from build123d import *

# Parameters (mm, degrees)
SKETCH1_R           = 1.625
SKETCH1_W           = 4
SKETCH1_H           = 10
BOSS_EXTRUDE1_DEPTH = 4


with BuildPart() as part:
    # Sketch1 → Boss-Extrude1 (new body)
    with BuildSketch(Plane(origin=(0, 0, 0), x_dir=(1, 0, 0), z_dir=(0, 1, 0))):
        Polygon((0, 0), (20, 0), (27.5, 0), (27.5, 4), (42.5, 4), (42.5, 0), (50, 0), (70, 0), (70, 26), (0, 26), align=None)
        with Locations((10, 19)):
            Circle(SKETCH1_R, mode=Mode.SUBTRACT)
        with Locations((60, 19)):
            Circle(SKETCH1_R, mode=Mode.SUBTRACT)
        with Locations((20, 16)):
            Rectangle(SKETCH1_W, SKETCH1_H, mode=Mode.SUBTRACT)
        with Locations((50, 16)):
            Rectangle(SKETCH1_W, SKETCH1_H, mode=Mode.SUBTRACT)
    extrude(amount=BOSS_EXTRUDE1_DEPTH)


solid = part.part
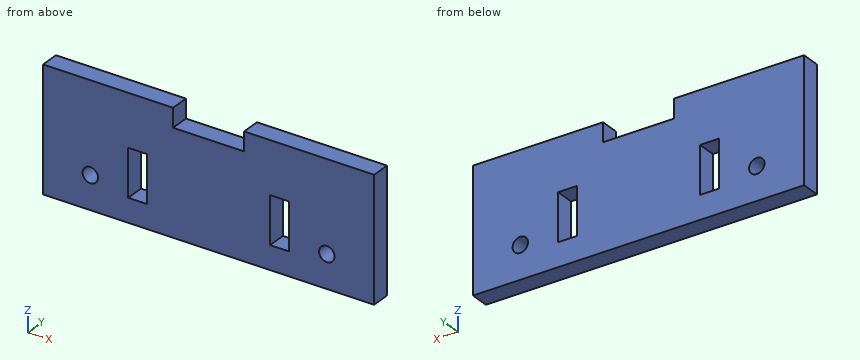
Source: CAD feature listing. Evaluate the final solid. Frame: model axes, mm. Coordinates: 2 decimals unless noted, no trailing zeros. Loops run counter-clockwise (first coordinate to the right, second up) from the corner with the lowest first, then second, coordinate; pieces in that order, holes last. Notation, with made-up numbers: (-33.75, -24) - (15.25, -24) arc R18 cw to (15.25, -7) - close; hole circle Ø8 at (-36, 0). An arc over 180 degrees is marked (long way). One line per item, written item: value. Start each with the question number.
1. Section B-B (y = 3.3). Return the cut outline in (x, z) (3 decimals).
2. Ray query, L1, parallel to X at y = 0.3, z = -15; L2, parallel to X at y = 2.45, z = -19 (3 decimals); L3, parallel to Z at x = 60, y = 2.7 (3 decimals). Return the intervals inside material, ascending.
3. Section A-A (z = -2.75). Return the cut outline in (x, y), and give its area (3 significant figures).
4. Contact query for a flat-ended pin moving along its axis: P1, Ø2, axis at x = 58, z = -3, coming from the -Y side. Output: stop coordinate, or through.
5. Section C-C (x = 60). Return the cut outline in (y, z) (3 decimals), and give its area (3 significant figures).
6. Section D-D (z = -18). Return the cut outline in (x, y), and give its area (3 significant figures).
Verdict:
1. outline: (0, -26) - (70, -26) - (70, 0) - (42.5, 0) - (42.5, -4) - (27.5, -4) - (27.5, 0) - (0, 0) - close; hole circle Ø3.25 at (10, -19); hole (18, -21) - (22, -21) - (22, -11) - (18, -11) - close; hole (48, -21) - (52, -21) - (52, -11) - (48, -11) - close; hole circle Ø3.25 at (60, -19)
2. L1: x = 0 to 18, 22 to 48, 52 to 70
2. L2: x = 0 to 8.375, 11.625 to 18, 22 to 48, 52 to 58.375, 61.625 to 70
2. L3: z = -26 to -20.625, -17.375 to 0
3. outline: (0, 0) - (27.5, 0) - (27.5, 4) - (0, 4) - close; (42.5, 0) - (70, 0) - (70, 4) - (42.5, 4) - close
3. area: 220 mm2
4. P1: stops at y = 0
5. outline: (0, -26) - (4, -26) - (4, -20.625) - (0, -20.625) - close; (0, -17.375) - (4, -17.375) - (4, 0) - (0, 0) - close
5. area: 91.0 mm2
6. outline: (0, 0) - (8.72, 0) - (8.72, 4) - (0, 4) - close; (11.28, 0) - (18, 0) - (18, 4) - (11.28, 4) - close; (22, 0) - (48, 0) - (48, 4) - (22, 4) - close; (52, 0) - (58.72, 0) - (58.72, 4) - (52, 4) - close; (61.28, 0) - (70, 0) - (70, 4) - (61.28, 4) - close
6. area: 228 mm2
